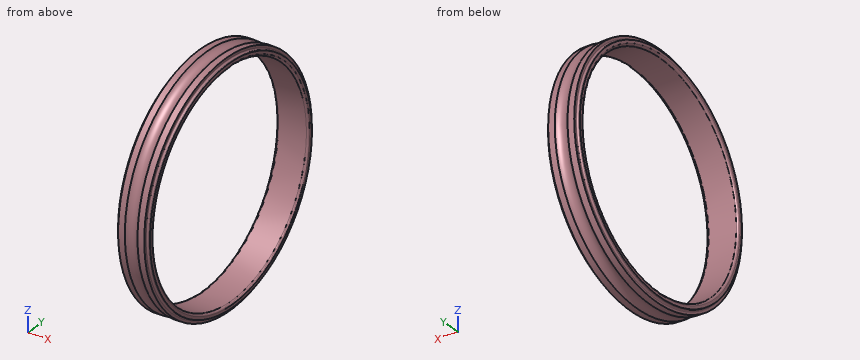
Solid Edge part; units mm, degrees
sketch "Sketch1" plane through (0, 0, 0) normal (0, 0, 1) x (1, 0, 0)
  arc A0 (0, 56) -> (1, 55) centre (1, 56) ccw
  line L0 (1, 55) -> (15, 55)
  arc A1 (15, 55) -> (16, 56) centre (15, 56) ccw
  line L1 (16, 56) -> (16, 59.167)
  arc A2 (16, 59.167) -> (15.667, 59.5) centre (15.667, 59.167) ccw
  line L2 (15.667, 59.5) -> (11.1721, 59.5)
  arc A3 (11.1721, 59.5) -> (4.8279, 59.5) centre (8, 62.5) cw
  line L3 (4.8279, 59.5) -> (0.333, 59.5)
  arc A4 (0.333, 59.5) -> (0, 59.167) centre (0.333, 59.167) ccw
  line L4 (0, 59.167) -> (0, 56)
revolve "RevolvedProtrusion1" add sketch "Sketch1" angle 360 about axis through (15, 0, 0) along (-1, 0, 0)
sketch "Sketch2" plane through (0, 0, 0) normal (0, 0, 1) x (1, 0, 0)
  line L0 (0, 57.5) -> (0.7268, 57.5)
  arc A0 (0.7268, 57.5) -> (1.4536, 58.2268) centre (0.7268, 58.2268) ccw
  line L1 (1.4536, 58.2268) -> (1.4536, 61.5)
  line L2 (1.4536, 61.5) -> (14.5464, 61.5)
  line L3 (14.5464, 61.5) -> (14.5464, 58.2268)
  arc A1 (14.5464, 58.2268) -> (15.2732, 57.5) centre (15.2732, 58.2268) ccw
  line L4 (15.2732, 57.5) -> (16, 57.5)
  line L5 (16, 57.5) -> (16, 63.5)
  line L6 (16, 63.5) -> (0, 63.5)
  line L7 (0, 63.5) -> (0, 57.5)
revolve "RevolvedCutout1" cut sketch "Sketch2" angle 360 about axis through (16, 0, 0) along (-1, 0, 0)
Model file for the job. Use its own axes, mm. Coordinates: 2 decimals unless noted, no trailing zeros. Loops run counter-clockwise (first coordinate to the right, second up) from the corner with the lowest first, then second, coordinate; pieces in that order, holes last. Notation, with made-up numbers: (-24.75, -18) - (31.25, -18) arc R9 ccw to (31.25, -14) - close; hole circle Ø1 at (0.5, 84). An arc over 180 degrees is marked (long way). Answer as a JSON object with one key per item and string values. Group by question number.
(1) Flat gauge pins, fed straight in: pin 1 (5 mm diameter, centred on x = 3, z = -15, fed in from +Y); pin 2 (1 mm diameter, centred on x = 12, y = 24, fed in from -Z); pin 3 (6 mm diameter, centred on x = 14, z = -32, fed in from +Y). Where does each tip first touch, or does it go through?
(2) Cut at C-C (x = 6.5). Give the cut face in (y, z), then the cut area to 3 significant figures.
(3) Cut at A-A (z = 0). Give the cut face in (x, y), then the cut area to 3 significant figures.
(4) Probe line 1 along Y through (x, z) = (9, 0); line 2 along Y through (x, z) = (7.25, 0). List the from-to ranges inside material, lowest first.
Geometry says:
{
 "1": {"pin 1": "stops at y = 58.17", "pin 2": "stops at z = -54.66", "pin 3": "stops at y = 51.95"},
 "2": {"outline": "circle Ø116.8 at (0, 0); hole circle Ø110 at (0, 0)", "area": "1,210 mm^2"},
 "3": {"outline": "(0, -57.5) - (0.73, -57.5) arc R0.73 cw to (1.45, -58.23) - (1.45, -59.5) - (4.83, -59.5) arc R4.37 cw to (11.17, -59.5) - (14.55, -59.5) - (14.55, -58.23) arc R0.73 cw to (15.27, -57.5) - (16, -57.5) - (16, -56) arc R1 ccw to (15, -55) - (1, -55) arc R1 ccw to (0, -56) - close; (0, 56) arc R1 ccw to (1, 55) - (15, 55) arc R1 ccw to (16, 56) - (16, 57.5) - (15.27, 57.5) arc R0.73 cw to (14.55, 58.23) - (14.55, 59.5) - (11.17, 59.5) arc R4.37 cw to (4.83, 59.5) - (1.45, 59.5) - (1.45, 58.23) arc R0.73 cw to (0.73, 57.5) - (0, 57.5) - close", "area": "120 mm^2"},
 "4": {"line 1": "y = -58.25 to -55, 55 to 58.25", "line 2": "y = -58.2 to -55, 55 to 58.2"}
}
